Geometry check sheet. Reference: drawing and pictorial views, mm from the part's lowest x, y, z. A direction names the side the tool comes from. Give positions to 0.01 mm unless a question says otherwise; leave off trailing zeros. Write each loop counter-clockwise with the first axis right and the second up, starting at its lowest first coordinate (ties: lowest second). Pieces come first, ordered by that corner, then holes. Notation, with made-up numbers: (67.5, 34.25) -> (121.5, 34.25) arc R23 cw to (121.5, 50.25) -> close; hole circle Ø9 at (76, 1). An arc over 180 degrees is marked (long way). Return JSON: item names as keys, results as strings.
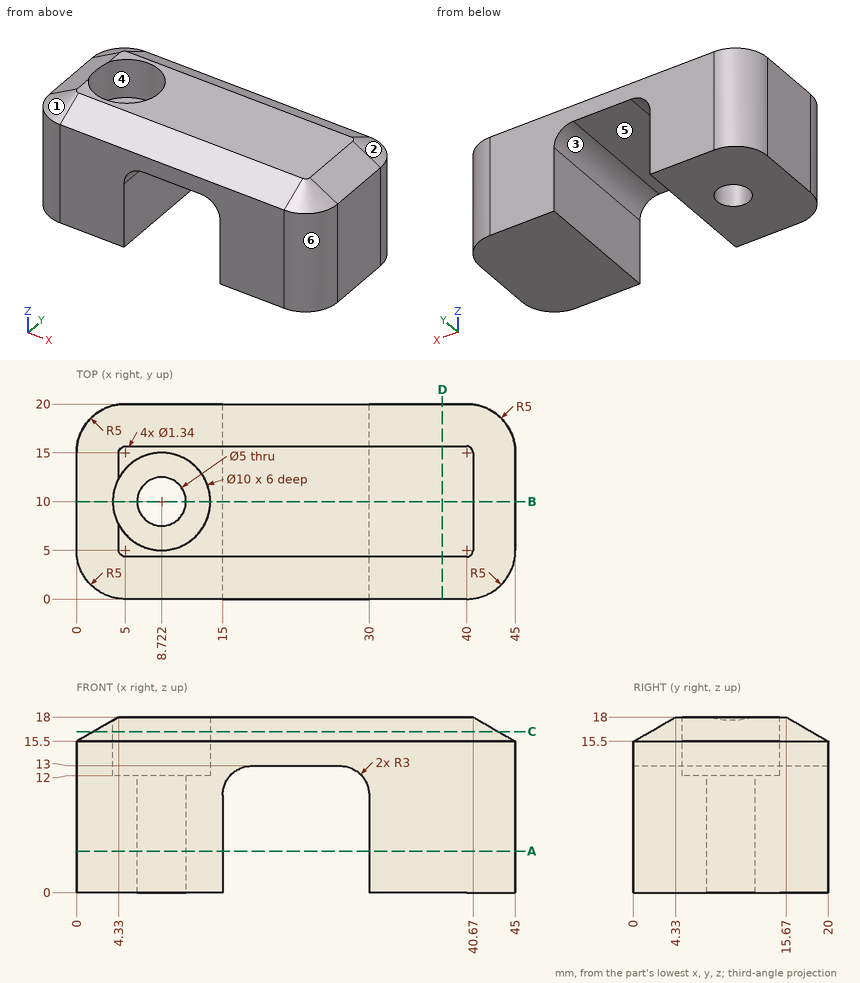
(1) Thickness scan on L1, parallel to X at y = 9.5, z = 2.5; L2, parallel to Y at x = 8.5, z = 5.75; L3, parallel to X at y = 10, z = 14.9. Record the ranges inside material, lowest first.
Reply:
{"L1": "0 to 6.27, 11.17 to 15, 30 to 45", "L2": "0 to 7.51, 12.49 to 20", "L3": "0 to 3.72, 13.72 to 45"}
(2) Cross-section at D-D on x = 37.5. Enter the section's corners in (y, z), then the cut area to 3 significant figures.
Reply:
{"outline": "(0, 0) -> (20, 0) -> (20, 15.5) -> (15.67, 18) -> (4.33, 18) -> (0, 15.5) -> close", "area": "349 mm^2"}
(3) Release check for a two-part mould opening along X. For the marked faces 1, 2 and 3 record: pulls with the +X half, pulls with the -X half, needs draft (parallel to the pull), parting line crosses it, or undercut.
Reply:
{"face 1": "pulls with the -X half", "face 2": "pulls with the +X half", "face 3": "undercut"}
(4) Cross-section at B-B on y = 10. Enter the section's corners in (x, z).
Reply:
{"outline": "(0, 0) -> (6.22, 0) -> (6.22, 12) -> (3.72, 12) -> (3.72, 17.65) -> (0, 15.5) -> close; (11.22, 0) -> (15, 0) -> (15, 10) arc R3 cw to (18, 13) -> (27, 13) arc R3 cw to (30, 10) -> (30, 0) -> (45, 0) -> (45, 15.5) -> (40.67, 18) -> (13.72, 18) -> (13.72, 12) -> (11.22, 12) -> close"}
(5) Cross-section at A-A on z = 4.25. Enter the section's corners in (x, y), then the cut area to 3 significant figures.
Reply:
{"outline": "(0, 5) arc R5 ccw to (5, 0) -> (15, 0) -> (15, 20) -> (5, 20) arc R5 ccw to (0, 15) -> close; (30, 0) -> (40, 0) arc R5 ccw to (45, 5) -> (45, 15) arc R5 ccw to (40, 20) -> (30, 20) -> close; hole circle Ø5 at (8.72, 10)", "area": "559 mm^2"}
(6) Depth check by flat-ended pin: pin 1 Ø10 at (x, y) = (22.5, 11) entering from -Z. Enter the tip coordinate at first touch or a pass-through.
Reply:
{"pin 1": "z = 12.96"}
(7) Cross-section at C-C on z = 16.5. Enter the section's corners in (x, y), then the cut area to 3 significant figures.
Reply:
{"outline": "(1.73, 5) arc R3.27 ccw to (5, 1.73) -> (40, 1.73) arc R3.27 ccw to (43.27, 5) -> (43.27, 15) arc R3.27 ccw to (40, 18.27) -> (5, 18.27) arc R3.27 ccw to (1.73, 15) -> close; hole circle Ø10 at (8.72, 10)", "area": "599 mm^2"}
(8) Set-up check for the marked faces 4, 5 and 6: record each of +Z, -Z, +X, -X, +Y, -Y from which the full face is reachable in a straight line by a thin tool's end or side.
Reply:
{"face 4": "+Z", "face 5": "-Z, +Y, -Y", "face 6": "+Z, -Z, +X, -Y"}
